```python
from build123d import *

# Parameters (mm, degrees)
F0_R          = 1.75
F1_DEPTH      = 3.5
F2_DEPTH      = 6
F0_W          = 1
F0_H          = 0.5
F3_DEPTH      = 1
F3_DEPTH_BACK = 3.5


with BuildPart() as f1:
    # F0 (on Top) → F1 (new body)
    with BuildSketch(Plane.XY):
        Polygon((3, 2.75), (3, 3), (-3, 3), (-3, 2.75), (-3, 2.25), (-3, -2.25), (-3, -2.75), (-3, -3), (3, -3), (3, -2.75), (3, -2.25), (3, 2.25), align=None)
        Circle(F0_R, mode=Mode.SUBTRACT)
    extrude(amount=F1_DEPTH)

    # F0 (on Top) → F2 (join)
    with BuildSketch(Plane.XY):
        Circle(F0_R)
    extrude(amount=F2_DEPTH)

    # F0 (on Top) → F3 (join, two sides)
    with BuildSketch(Plane.XY) as f3_sk:
        with Locations((-3.5, -2.5)):
            Rectangle(F0_W, F0_H)
        with Locations((-3.5, 2.5)):
            Rectangle(F0_W, F0_H)
        with Locations((3.5, 2.5)):
            Rectangle(F0_W, F0_H)
        with Locations((3.5, -2.5)):
            Rectangle(F0_W, F0_H)
    extrude(amount=F3_DEPTH)
    extrude(f3_sk.sketch, amount=-F3_DEPTH_BACK)


solid = f1.part
```
For this review, take the finished solid that the model builds, in its own axes (mm). A direction names the side the tool comes from. Round coordinates to 2 decimals unless told otherwise and drop trailing zeros. Write each loop counter-clockwise with the first axis right and the second up, starting at its lowest first coordinate (ties: lowest second). Pieces come first, ordered by that corner, then holes. Notation, with made-up numbers: M 2.25,77 L 43.25,77 A31 ccw 43.25,112 Z; hole C -12.5,31.5 d6. An arc over 180 degrees is marked long. One line per item, written item: value. Start each with the question number.
(1) We need section D-D (x = 0). Give the boundary of the cut face in (y, z).
(2) We need section B-B (x = 3.75). Give the boundary of the cut face in (y, z).
(3) We need section A-A (z = -2). Give the boundary of the cut face in (x, y).
(4) Insertion check: pin 1 (0.5 mm diameter, centred on x = 3.5, z = -2, fed in from -Y); pin 2 (1.1 mm diameter, centred on x = 3.5, z = -1, fed in from +Y); pin 3 (1 mm diameter, centred on y = -0.5, z = 2.5, fed in from +X). Each pin has a flat end and moves straight along its axis. Give the tip position at first contact, or say it passes through.
(5) Machinability: for faces 1 (the flat face through (0, 0, 0)), 2 (the flat face through (-3.5, -2.25, -1.2)), 3 (the flat face through (3.5, -2.75, -1.3)), 4 (the cylindrical face through (1.617, -0.67, 4.732)), which of the approach directions +Z, -Z, +X, -X, +Y, -Y give a long, thin tool a straight path to every point of the face, cutting with its end or side? Answer none if there is none.
(6) We need section C-C (y = -2.45). Give the boundary of the cut face in (x, z).
(7) The part is to be moulded in two halves that separate along Y. For faces 5 (the flat face through (3.5, -2.25, -1.3)), 6 (the flat face through (0, -3, 2)), 7 (the flat face through (3.5, 2.75, -1.3)), say which applies: released by +Y, released by -Y, zero draft, split by the parting line, or undercut.
(8) Wall thickness on line 1 (Y direction, x = -3.5, z = -1.5); line 2 (Z direction, x = -1.5, y = 0.05); line 3 (Z direction, x = -2.5, y = -0.7): over which ranges is each line inside the solid? List them lowest first.
Result:
1. outline: M -3,0 L 3,0 L 3,3.5 L 1.75,3.5 L 1.75,6 L -1.75,6 L -1.75,3.5 L -3,3.5 Z
2. outline: M -2.75,-3.5 L -2.25,-3.5 L -2.25,1 L -2.75,1 Z; M 2.25,-3.5 L 2.75,-3.5 L 2.75,1 L 2.25,1 Z
3. outline: M -4,-2.75 L -3,-2.75 L -3,-2.25 L -4,-2.25 Z; M -4,2.25 L -3,2.25 L -3,2.75 L -4,2.75 Z; M 3,-2.75 L 4,-2.75 L 4,-2.25 L 3,-2.25 Z; M 3,2.25 L 4,2.25 L 4,2.75 L 3,2.75 Z
4. pin 1: y = -2.75
4. pin 2: y = 2.75
4. pin 3: x = 3
5. face 1: -Z, +Y, -Y
5. face 2: +Z, -Z, -X
5. face 3: +Z, -Z, +X, -Y
5. face 4: +Z
6. outline: M -4,-3.5 L -3,-3.5 L -3,0 L 3,0 L 3,-3.5 L 4,-3.5 L 4,1 L 3,1 L 3,3.5 L -3,3.5 L -3,1 L -4,1 Z
7. face 5: undercut
7. face 6: released by -Y
7. face 7: released by +Y
8. line 1: -2.75 to -2.25, 2.25 to 2.75
8. line 2: 0 to 6
8. line 3: 0 to 3.5
